Work out the finished part from the listing and answer in its coordinate system (mm). Coordinates: 2 decimals unless noted, no trailing zeros. Loops run counter-clockwise (first coordinate to the right, second up) from the corner with the lowest first, then second, coordinate; pieces in that order, holes last. Notation, with made-up numbers: M 43.25,43 L 48.25,43 A30 cw 48.25,74 Z; hole C -27.75,-26 d6. An arc over 180 degrees is marked long. Write each question's results on one line, items separated by ' | '.
```python
from build123d import *

# Parameters (mm, degrees)
SKETCH1_W                    = 482.6
SKETCH1_H                    = 175.006
BASE_FLANGE_DEPTH            = 3.175
SKETCH2_W                    = 165.2016
SKETCH2_H                    = 124.6886
CUT_EXTRUDE1_DEPTH           = 514.361413296
F_1_8_0_125_DIAMETER_HOLE1_D = 3.175
LPATTERN1_COUNT              = 2
LPATTERN1_PITCH              = 116.0018
LPATTERN1_COUNT_DIR2         = 2
LPATTERN1_PITCH_DIR2         = 196.596
CUT_EXTRUDE2_DEPTH           = 514.361413296
LPATTERN2_COUNT              = 3
LPATTERN2_PITCH              = 25.4
SKETCH5_R                    = 3.175
CUT_EXTRUDE3_DEPTH           = 514.361413296
LPATTERN3_COUNT              = 2
LPATTERN3_PITCH              = 408.8384
LPATTERN3_COUNT_DIR2         = 2
LPATTERN3_PITCH_DIR2         = 88.9


# Sheet-metal steps are written as plain solids
with BuildPart() as part:
    # Sketch1 → Base-Flange (new body)
    with BuildSketch(Plane.XY):
        with Locations((241.3, 87.503)):
            Rectangle(SKETCH1_W, SKETCH1_H)
    extrude(amount=BASE_FLANGE_DEPTH)

    # Sketch2 → Cut-Extrude1 (cut, through all)
    with BuildSketch(Plane.XY.offset(3.175)):
        with Locations((158.8008, 87.503)):
            Rectangle(SKETCH2_W, SKETCH2_H)
    extrude(amount=-CUT_EXTRUDE1_DEPTH, mode=Mode.SUBTRACT)

    # 1/8 (0.125) Diameter Hole1 (through all)
    with Locations(Plane(origin=(60.5028, 29.5021, 3.175), x_dir=(1, 0, 0), z_dir=(0, 0, 1))):
        with Locations((0, 0)):
            f_1_8_0_125_diameter_hole1 = Hole(F_1_8_0_125_DIAMETER_HOLE1_D / 2)

    # LPattern1: 1_8 _0.125_ Diameter Hole1 2 × 2
    with Locations(*[(j * LPATTERN1_PITCH_DIR2, i * LPATTERN1_PITCH, 0) for i in range(LPATTERN1_COUNT) for j in range(LPATTERN1_COUNT_DIR2) if (i, j) != (0, 0)]):
        add(f_1_8_0_125_diameter_hole1, mode=Mode.SUBTRACT)

    # Sketch4 → Cut-Extrude2 (cut, through all)
    with BuildSketch(Plane.XY.offset(3.175)):
        with BuildLine():
            Line((296.1513, 73.343363249), (296.1513, 78.574036751))
            ThreePointArc((296.1513, 78.574036751), (287.4645, 75.9587), (296.1513, 73.343363249))
        make_face()
    cut_extrude2 = extrude(amount=-CUT_EXTRUDE2_DEPTH, mode=Mode.SUBTRACT)

    # LPattern2: Cut-Extrude2 ×3
    with Locations(*[(0, i * LPATTERN2_PITCH, 0) for i in range(1, LPATTERN2_COUNT)]):
        add(cut_extrude2, mode=Mode.SUBTRACT)

    # Sketch5 → Cut-Extrude3 (cut, through all)
    with BuildSketch(Plane.XY.offset(3.175)):
        with Locations((292.2016, 39.3827)):
            Circle(SKETCH5_R)
    extrude(amount=-CUT_EXTRUDE3_DEPTH, mode=Mode.SUBTRACT)

    # Sketch6 → #40 (0.098) Diameter Hole1 (revolve, cut)
    with BuildSketch(Plane(origin=(36.8808, 43.053, 3.175), x_dir=(0, -1, 0), z_dir=(1, 0, 0))):
        Polygon((0, 0), (0, 4.192530181), (1.778, 3.1242), (1.778, 0), align=None)
    f_40_0_098_diameter_hole1 = revolve(axis=Axis((36.8808, 43.053, 9.525), (0, 0, -1)), mode=Mode.SUBTRACT)

    # LPattern3: 40 _0.098_ Diameter Hole1 2 × 2
    with Locations(*[(i * LPATTERN3_PITCH, j * LPATTERN3_PITCH_DIR2, 0) for i in range(LPATTERN3_COUNT) for j in range(LPATTERN3_COUNT_DIR2) if (i, j) != (0, 0)]):
        add(f_40_0_098_diameter_hole1, mode=Mode.SUBTRACT)


solid = part.part
```
1) Find section C-C, the plane z = 2.1. Give the number of separate pieces and of enclosed holes in the cut face, and give its area (3 significant figures).
Check result:
separate pieces: 1 | enclosed holes: 13 | area: 63,600 mm^2
2) For a pull along Y with two mould halves and no side action, classify faces 1 (the face through (287.468, 126.928, 1.61)), 2 (the face through (292, 89, 0)) as released by +Y, released by -Y, zero draft, split by the parting line, or undercut.
Check result:
face 1: undercut | face 2: zero draft
3) Straight lines are drawn through the part: probe 1 along X at (y, z) = (146, 2); probe 2 along Y at (x, z) = (240.5, 1.5); probe 3 along X at (y, z) = (87, 2.6). For each, find the intervals that lie inside material, in ascending order. Write a range as [from, to].
Check result:
probe 1: [0, 58.99], [62.01, 76.2], [241.4, 255.59], [258.61, 482.6] | probe 2: [0, 25.16], [149.85, 175.01] | probe 3: [0, 76.2], [241.4, 482.6]
4) Find section B-B, the plane x = 142. Give the vertices of the cut face in (y, z) (3 decimals), and give its area (3 significant figures).
Check result:
outline: M 0,0 L 25.159,0 L 25.159,3.175 L 0,3.175 Z; M 149.847,0 L 175.006,0 L 175.006,3.175 L 149.847,3.175 Z | area: 160 mm^2
5) Find section A-A, the plane y = 60. Give the vertices of the cut face in (x, z) (3 decimals).
Check result:
outline: M 0,0 L 76.2,0 L 76.2,3.175 L 0,3.175 Z; M 241.402,0 L 482.6,0 L 482.6,3.175 L 241.402,3.175 Z
